Autodesk Inventor part; units mm, degrees
ref_plane "YZ Plane" through (0, 0, 0) normal (1, 0, 0) x (0, 1, 0)
ref_plane "XZ Plane" through (0, 0, 0) normal (0, 1, 0) x (-1, 0, 0)
ref_plane "XY Plane" through (0, 0, 0) normal (0, 0, 1) x (1, 0, 0)
sketch "Sketch1" plane through (0, 0, 0) normal (0, 0, 1) x (1, 0, 0)
  line L0 (0, 3.5) -> (0, -7)
  line L1 (0, 0) -> (4.25, 0) construction
  arc A0 (4.25, 0.2391) -> (0, 3.5) centre (0, -0.9) ccw
  line L2 (4.25, 0) -> (2.5, 0)
  line L3 (2.5, 0) -> (2.5, -7)
  line L4 (2.5, -7) -> (0, -7)
  line L5 (4.25, 0) -> (4.25, 0.2391)
  dimension "d1" = 3.5
  dimension "d2" = 4.4
  dimension "d3" = 5
  dimension "d4" = 7
  dimension "d25" = 8.5
revolve "Вращение1" add sketch "Sketch1" angle 360 about axis through (0, 3.5, 0) along (0, -1, 0)
sketch "Sketch2" plane through (0, 0, 0) normal (0, 0, 1) x (1, 0, 0)
  line L0 (-0.6, 3.5) -> (0.6, 3.5)
  line L1 (0.6, 3.5) -> (0.6, 1.3)
  line L2 (0.6, 1.3) -> (-0.6, 1.3)
  line L3 (-0.6, 1.3) -> (-0.6, 3.5)
  line L4 (0, 0) -> (0, 3.5)
  arc A0 (4.25, 0.2391) -> (-4.25, 0.2391) centre (0, -0.9) ccw construction
  dimension "d6" = 1.3
  dimension "d7" = 1.2
extrude "Выдавливание1" cut sketch "Sketch2" along normal through all both and the other way through all
thread "Резьба1"
fillet "Сопряжение1" radius 0.3333 1 edges at (-2.5, 0, 0)
chamfer "Фаска1" distance 0.3333 angle 45 1 edges at (-2.5, -7, 0)
equation "\"d6\" = w"
equation "\"d7\" = n"
equation "\"d10\" = b"
equation "\"d12\" = c_"
equation "\"d13\" = c_"
equation "\"d1\" = k"
equation "\"d2\" = R1"
equation "\"d3\" = d_"
equation "\"d4\" = l_"
equation "\"d25\" = D"
equation "\"d_\" = 5"
equation "\"D\" = 8.5"
equation "\"k\" = 3.5"
equation "\"l_\" = 7"
equation "\"b\" = 7"
equation "\"n\" = 1.2"
equation "\"w\" = 1.3"
equation "\"c_\" = 0.0666667 * d_"
equation "\"R1\" = 4.4"
equation "\"G\" = 0"
properties part number "Винт A.M5-6gx7 ГОСТ 17473-80" material "Сталь, мягкая"
Geometry: final body of the model. Coordinates: model frame, mm. A direction names the side the tool comes from. Give positions to 0.01 mm unless a question says otherwise; leave off trailing zeros. Write each loop counter-clockwise with the first axis right and the second up, starting at its lowest first coordinate (ties: lowest second). Pieces come first, ordered by that corner, then holes.
1. Reachability of faces 1 (the flat face through (1, 0, -3)), 2 (the flat face through (0, 1.3, 0)) from +Z, -Z, +X, -X, +Y, -Y: full face, straight path, thin tool, end or side. Return the list, or none.
2. Pin query (flat end, axial travel): P1, Ø3, axis at x = -3.5, z = -3, coming from the -Y side; P2, Ø1.1, axis at y = 3, z = -1.5, coming from the -X side; P3, Ø0.6, axis at x = 0, z = -1, coming from the +Y side. Return the tip coordinate at first contact, or that it passes through.
3. Line query: probe 1 along X at (y, z) = (-6.5, -1.25); probe 2 along X at (y, z) = (1.5, -1); probe 3 along Y at (x, z) = (0.5, -1). Output: solid intervals per line, ascending.
4. Draft query along X for faces 3 (the cylindrical face through (-0.54, -3.54, -2.44)), 4 (the flat face through (0, -7, 0)), 5 (the flat face through (0.6, 2, 0)). Return one class per face: released by +X, released by -X, zero draft, split by the parting line, or undercut.
5. Section query A-A, the plane y = -5.5. Return loops of the section in (x, z), then the cut area to 3 significant figures.
Computed:
1. face 1: -Y
1. face 2: +Z, -Z, +Y
2. P1: stops at y = 0
2. P2: stops at x = -2.49
2. P3: stops at y = 1.3
3. probe 1: x = -2.17 to 2.17
3. probe 2: x = -3.55 to -0.6, 0.6 to 3.55
3. probe 3: y = -7 to 1.3
4. face 3: split by the parting line
4. face 4: zero draft
4. face 5: undercut
5. outline: circle Ø5 at (0, 0)
5. area: 19.6 mm2
